Could you check a few things on this model? Use its own coordinates, in mm. A direction names the side the tool comes from. Give positions to 0.01 mm unless a question says otherwise; leave off trailing zeros. Loops run counter-clockwise (first coordinate to the right, second up) from the corner with the lowest first, then second, coordinate; pieces in that order, holes last. Notation, with made-up numbers: (4, 10.25) - (60, 10.25) arc R35 ccw to (60, 48.25) - close; hole circle Ø9 at (15, 9.5). An arc over 180 degrees is marked (long way). Write each question's results on one line, items separated by ' | '. Start each with the question number.
(1) I need wall thicknesses on line 1 (Y direction, x = 0, z = 5.5); line 2 (Y direction, x = -0.75, z = 53); line 3 (X direction, y = -0.25, z = 217.5). Which ranges of each line are inside material? Lowest first, please.
(2) For pin 1 (4 mm diameter, centred on x = 3, z = 162, fed in from +Y); pin 2 (2 mm diameter, centred on y = -2, z = 269.5, fed in from +X); pin 3 (12 mm diameter, centred on x = -8.5, z = 213.5, fed in from -Y); pin 4 (17.5 mm diameter, centred on x = 0, y = 0, fed in from -Z), each with a flat end and sliding along its axis, tell me the tip position at first contact or that it passes through.
(3) Suppose I cut it at B-B (y = 5). Please give me the cut outline in (x, z), and give its area (3 significant figures).
(4) Suppose I cut it at A-A (x = 0). Please give me the cut outline in (y, z), and give its area (3 significant figures).
(5) If we mould it in two halves opening along X, with no side actions, what happens to faces 1 (the face through (-0.1, 13.4, 0)), 2 (the face through (10.316, -7.91, 3.451)), 3 (the face through (-14.985, 0.66, 152.83))? For each: released by +X, released by -X, zero draft, split by the parting line, or undercut.
(6) Suppose I cut it at C-C (z = 19.5). Please give me the cut outline in (x, y).
(7) On a 3-axis mill with a long thin cutter (end or side, diameter ignored), from which of +Z, -Z, +X, -X, +Y, -Y can I reach the whole of each face in a straight line? I mean faces 4 (the face through (-7, -8, 7)), 5 (the face through (-5, 10, 310)), 6 (the face through (-2.38, -10.74, 304.08)). Say none if no direction works.
from build123d import *

# Parameters (mm, degrees)
ESQUISSE1_R             = 15
ESQUISSE1_R_2           = 10
BOSS_EXTRU_1_DEPTH      = 310
ESQUISSE2_R             = 13
ESQUISSE2_R_2           = 10
ENL_V_MAT_EXTRU_1_DEPTH = 7
ESQUISSE3_R             = 11
ESQUISSE3_R_2           = 10
ENL_V_MAT_EXTRU_2_DEPTH = 12


with BuildPart() as part:
    # Esquisse1 → Boss.-Extru.1 (new body)
    with BuildSketch(Plane.XY):
        Circle(ESQUISSE1_R)
        Circle(ESQUISSE1_R_2, mode=Mode.SUBTRACT)
    extrude(amount=BOSS_EXTRU_1_DEPTH)

    # Esquisse2 → Enlèv. mat.-Extru.1 (cut)
    with BuildSketch(Plane(origin=(0, 0, 0), x_dir=(-1, 0, 0), z_dir=(0, 0, -1))):
        Circle(ESQUISSE2_R)
        Circle(ESQUISSE2_R_2, mode=Mode.SUBTRACT)
    extrude(amount=-ENL_V_MAT_EXTRU_1_DEPTH, mode=Mode.SUBTRACT)

    # Esquisse3 → Enlèv. mat.-Extru.2 (cut)
    with BuildSketch(Plane.XY.offset(310)):
        Circle(ESQUISSE3_R)
        with Locations(Location((0, 0, 0), (0, 0, 180))):  # turned: the seam where the file's is
            Circle(ESQUISSE3_R_2, mode=Mode.SUBTRACT)
    extrude(amount=-ENL_V_MAT_EXTRU_2_DEPTH, mode=Mode.SUBTRACT)


solid = part.part
Output values:
1) line 1: -15 to -13, 13 to 15 | line 2: -14.98 to -9.97, 9.97 to 14.98 | line 3: -15 to -10, 10 to 15
2) pin 1: y = 14.97 | pin 2: x = 14.97 | pin 3: y = -14.79 | pin 4: through
3) outline: (-14.14, 0) - (-12, 0) - (-12, 7) - (-8.66, 7) - (-8.66, 298) - (-9.8, 298) - (-9.8, 310) - (-14.14, 310) - close; (8.66, 7) - (12, 7) - (12, 0) - (14.14, 0) - (14.14, 310) - (9.8, 310) - (9.8, 298) - (8.66, 298) - close | area: 3,320 mm2
4) outline: (-15, 0) - (-13, 0) - (-13, 7) - (-10, 7) - (-10, 298) - (-11, 298) - (-11, 310) - (-15, 310) - close; (10, 7) - (13, 7) - (13, 0) - (15, 0) - (15, 310) - (11, 310) - (11, 298) - (10, 298) - close | area: 3,030 mm2
5) face 1: zero draft | face 2: undercut | face 3: split by the parting line
6) outline: circle Ø30 at (0, 0); hole circle Ø20 at (0, 0)
7) face 4: -Z | face 5: +Z, +X, -X, +Y, -Y | face 6: +Z
